from build123d import *

# Parameters (mm, degrees)
BOSS_EXTRUDE1_DEPTH = 215.9
FILLET2_R           = 1.27
CUT_EXTRUDE2_START  = 6.35
CUT_EXTRUDE2_DEPTH  = 203.2


with BuildPart() as part:
    # Sketch4 → Boss-Extrude1 (new body)
    with BuildSketch(Plane(origin=(0, 0, 0), x_dir=(1, 0, 0), z_dir=(0, 1, 0))):
        with BuildLine():
            Line((-28.9052, 0), (-38.1, 0))
            Line((-38.1, 0), (-46.99, -8.89))
            Line((-46.99, -8.89), (-38.1, -8.89))
            Line((-38.1, -8.89), (-37.04831845, -8.89))
            ThreePointArc((-37.04831845, -8.89), (4.475995255, -37.836166118), (38.1, 0))
            Line((38.1, 0), (28.9052, 0))
            ThreePointArc((28.9052, 0), (0, -28.9052), (-28.9052, 0))
        make_face()
    extrude(amount=BOSS_EXTRUDE1_DEPTH)

    # Fillet2
    fillet2_edges = [part.edges().sort_by_distance(p)[0] for p in [
        (-46.99, 107.95, 8.89),
    ]]
    fillet(fillet2_edges, radius=FILLET2_R)

    # Sketch6 → Cut-Extrude2 (cut)
    with BuildSketch(Plane(origin=(0, 0, 0), x_dir=(1, 0, 0), z_dir=(0, 1, 0)).offset(CUT_EXTRUDE2_START)):
        with BuildLine():
            ThreePointArc((-35.802288852, -13.030967461), (0, -38.1), (35.802288852, -13.030967461))
            ThreePointArc((35.802288852, -13.030967461), (29.90974259, -15.778706909), (27.162003142, -9.886160647))
            ThreePointArc((27.162003142, -9.886160647), (0, -28.9052), (-27.162003142, -9.886160647))
            ThreePointArc((-27.162003142, -9.886160647), (-29.90974259, -15.778706909), (-35.802288852, -13.030967461))
        make_face()
    extrude(amount=CUT_EXTRUDE2_DEPTH, mode=Mode.SUBTRACT)


solid = part.part
CAD build for the part. Positions are in the model's coordinates, mm. Give positions to 0.01 mm unless a question says otherwise; leave off trailing zeros. Loops run counter-clockwise (first coordinate to the right, second up) from the corner with the lowest first, then second, coordinate; pieces in that order, holes last. Notation, with made-up numbers: M 4,82 L 47,82 A25 ccw 47,108 Z; hole C -30,67 d8. An arc over 180 degrees is marked long. One line per question, with ' | ' between items. Start each with the question number.
1. Probe L1, parallel to Y at x = -29, z = 22; L2, parallel to X at y = 133, z = 10.5; L3, parallel to X at y = 177.5, z = 5.5. List the from-to ranges inside material, lowest first. Write a range as from..to.
2. Flat gauge pins, fed straight in: pin 1 (3 mm diameter, centred on x = 22, z = 23.5, fed in from -Y); pin 2 (5.5 mm diameter, centred on x = -40, y = 75, fed in from +Z); pin 3 (10 mm diameter, centred on x = -30, z = 32.5, fed in from -Y). Where does each tip first touch, or does it go through?
3. Saw through at C-C on z = 33.5. Give the cut face in (x, y).
4. Saw through at A-A on x = 0. Give the cut face in (y, z).
5. Saw through at B-B on z = 22. Give the cut face in (x, y), plus the area to 3 significant figures.
6. Two-plate mould, pull along Y, no slides. Class faces 1 (the face through (-0.2, 209.55, 29.2)), 2 (the face through (-4, 215.9, 29)), 3 (the face through (-29.815, 106.528, 15.743)), 4 (the face through (-41, 106, 8.89)): pulls with the +Y half, pulls with the -Y half, needs draft (parallel to the pull), parting line crosses it, or undercut.
Result sheet:
1) L1: y = 0..6.35, 209.55..215.9 | L2: x = -36.62..-26.99, 26.99..36.62 | L3: x = -43.6..-28.38, 28.38..37.7
2) pin 1: stops at y = 0 | pin 2: stops at z = 8.89 | pin 3: passes through
3) outline: M -18.15,0 L 18.15,0 L 18.15,6.35 L -18.15,6.35 Z; M -18.15,209.55 L 18.15,209.55 L 18.15,215.9 L -18.15,215.9 Z
4) outline: M 0,28.91 L 6.35,28.91 L 6.35,38.1 L 0,38.1 Z; M 209.55,28.91 L 215.9,28.91 L 215.9,38.1 L 209.55,38.1 Z
5) outline: M -31.11,0 L -18.75,0 L -18.75,6.35 L -31.11,6.35 Z; M -31.11,209.55 L -18.75,209.55 L -18.75,215.9 L -31.11,215.9 Z; M 18.75,0 L 31.11,0 L 31.11,6.35 L 18.75,6.35 Z; M 18.75,209.55 L 31.11,209.55 L 31.11,215.9 L 18.75,215.9 Z | area: 314 mm^2
6) face 1: undercut | face 2: pulls with the +Y half | face 3: undercut | face 4: needs draft
